```python
from build123d import *

# Parameters (mm, degrees)
EXTRUDE_2_DEPTH     = 10
SKETCH_2_R          = 10
CUT_EXTRUDE_1_DEPTH = 10
SKETCH_3_R          = 10
CUT_EXTRUDE_2_DEPTH = 10


with BuildPart() as part:
    # Эскиз1 → Бобышка-Вытянуть2 (new body)
    with BuildSketch(Plane.XY):
        with BuildLine():
            Line((0, 0), (-100, 0))
            ThreePointArc((-100, 0), (-115, 15), (-100, 30))
            Line((-100, 30), (0, 30))
            ThreePointArc((0, 30), (15, 15), (0, 0))
        make_face()
    extrude(amount=EXTRUDE_2_DEPTH)

    # Эскиз2 → Вырез-Вытянуть1 (cut)
    with BuildSketch(Plane(origin=(0, 0, 0), x_dir=(-1, 0, 0), z_dir=(0, 0, -1))):
        with Locations((0, 15)):
            Circle(SKETCH_2_R)
        with Locations((100, 15)):
            Circle(SKETCH_2_R)
    extrude(amount=-CUT_EXTRUDE_1_DEPTH, mode=Mode.SUBTRACT)

    # Эскиз3 → Вырез-Вытянуть2 (cut)
    with BuildSketch(Plane(origin=(0, 0, 0), x_dir=(-1, 0, 0), z_dir=(0, 0, -1))):
        with Locations((50, 15)):
            Circle(SKETCH_3_R)
    extrude(amount=-CUT_EXTRUDE_2_DEPTH, mode=Mode.SUBTRACT)


solid = part.part
```
Design review of the part built by this model. Coordinates are the model's own, in mm. Coordinates: 2 decimals unless noted, no trailing zeros. Write each loop counter-clockwise with the first axis right and the second up, starting at its lowest first coordinate (ties: lowest second). Pieces come first, ordered by that corner, then holes.
1) Insertion check: pin 1 (1.5 mm diameter, centred on y = 16.5, z = 2.5, fed in from -X); pin 2 (1 mm diameter, centred on y = 25, z = 6, fed in from -X); pin 3 (3 mm diameter, centred on y = 7, z = 3, fed in from +X). Each pin has a flat end and moves straight along its axis. Give the tip position at first contact, or say it passes through.
2) Add section C-C (z = 8). Write out the cut boundary in (x, y).
3) Mouldability with a two-part tool opening along X and no side actions: class faces 1 (the cylindrical face through (-92.63, 21.76, 4.93)), 2 (the cylindrical face through (-115, 15, 5)), 3 (the flat face through (-49.1, 25.2, 10)), 4 (the cylindrical face through (15, 15, 5)) as +X half, -X half, draft (parallel to the pull), parting line (faces both ways), or undercut.
4) Add section B-B (x = -50). Write out the cut boundary in (y, z), plus the area to 3 significant figures.
5) Add section A-A (y = 15). Write out the cut boundary in (x, z).
6) Add section D-D (y = 23). Write out the cut boundary in (x, z), plus the area to 3 significant figures.
7) To check wall thickness, follow L1, parallel to X at y = 20.5, z = 8.5; L2, parallel to X at y = 17, z = 1.75; L3, parallel to Y at x = -50, z = 7.25. State the ranges of each line that lie inside material, in increasing order.
Check result:
1. pin 1: stops at x = -114.98
1. pin 2: stops at x = -111.61
1. pin 3: stops at x = 13.52
2. outline: (-100, 0) - (0, 0) arc R15 ccw to (0, 30) - (-100, 30) arc R15 ccw to start; hole circle Ø20 at (-100, 15); hole circle Ø20 at (-50, 15); hole circle Ø20 at (0, 15)
3. face 1: undercut
3. face 2: -X half
3. face 3: draft
3. face 4: +X half
4. outline: (0, 0) - (5, 0) - (5, 10) - (0, 10) - close; (25, 0) - (30, 0) - (30, 10) - (25, 10) - close
4. area: 100 mm2
5. outline: (-115, 0) - (-110, 0) - (-110, 10) - (-115, 10) - close; (-90, 0) - (-60, 0) - (-60, 10) - (-90, 10) - close; (-40, 0) - (-10, 0) - (-10, 10) - (-40, 10) - close; (10, 0) - (15, 0) - (15, 10) - (10, 10) - close
6. outline: (-112.69, 0) - (-106, 0) - (-106, 10) - (-112.69, 10) - close; (-94, 0) - (-56, 0) - (-56, 10) - (-94, 10) - close; (-44, 0) - (-6, 0) - (-6, 10) - (-44, 10) - close; (6, 0) - (12.69, 0) - (12.69, 10) - (6, 10) - close
6. area: 894 mm2
7. L1: x = -113.96 to -108.35, -91.65 to -58.35, -41.65 to -8.35, 8.35 to 13.96
7. L2: x = -114.87 to -109.8, -90.2 to -59.8, -40.2 to -9.8, 9.8 to 14.87
7. L3: y = 0 to 5, 25 to 30
